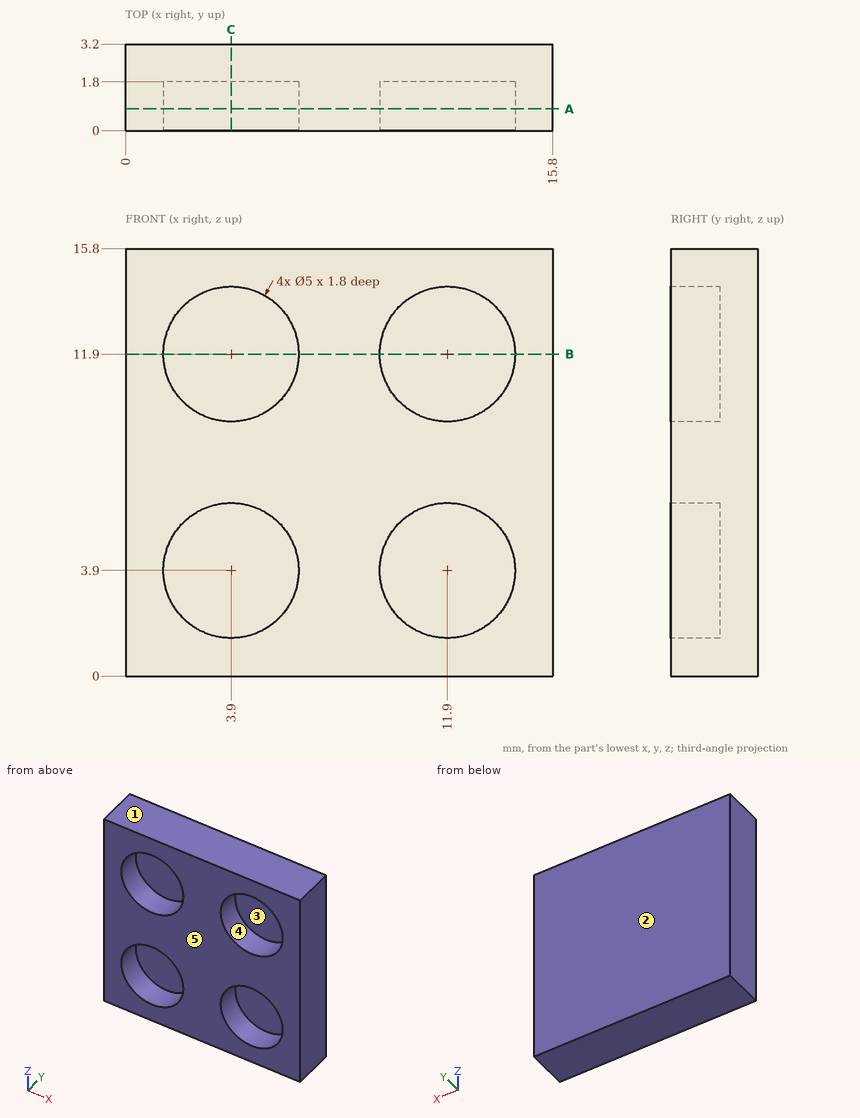
Study the drawing (mm; zero at the part's minimum x, y, z) and answer. A direction names the side the tool comes from. Round coordinates to 2 decimals unless told otherwise and drop trailing zeros. Loops run counter-clockwise (first coordinate to the right, second up) from the corner with the lowest first, then second, coordinate; pieces in that order, holes last.
Q1. Which of the six approach directions +Z, -Z, +X, -X, +Y, -Y give full straight-line access (tool end or side, diameter ignored) to the marked faces 4 and 5?
Q2. Given pin 1 Ø1.5 at (x, z) = (12, 13) entering from -Y, flat-ended and moving along its own axis, determine where the tip first touches the part or whether it passes through.
Q3. Find the intervals of material crossed by line 1 (X direction, y = 1, z = 11.9); line 2 (X direction, y = 1.4, z = 13) (3 decimals), in increasing order.
Q4. Section C-C, the plane x = 3.9 is taken. Determine the outline of the cut face in (y, z).
Q5. For a pull along Z with two mould halves and no side action, classify the marked faces 1, 2 and 3 as released by +Z, released by -Z, zero draft, split by the parting line, or undercut.
Q6. Section B-B, the plane z = 11.9 is taken. Determine the outline of the cut face in (x, y).
Q7. Section A-A, the plane y = 0.8 is taken. Determine the outline of the cut face in (x, z), then the cut area to 3 significant figures.
Completed:
1. face 4: -Y
1. face 5: +Z, -Z, +X, -X, -Y
2. pin 1: stops at y = 1.8
3. line 1: x = 0 to 1.4, 6.4 to 9.4, 14.4 to 15.8
3. line 2: x = 0 to 1.655, 6.145 to 9.655, 14.145 to 15.8
4. outline: (0, 0) - (3.2, 0) - (3.2, 15.8) - (0, 15.8) - (0, 14.4) - (1.8, 14.4) - (1.8, 9.4) - (0, 9.4) - (0, 6.4) - (1.8, 6.4) - (1.8, 1.4) - (0, 1.4) - close
5. face 1: released by +Z
5. face 2: zero draft
5. face 3: undercut
6. outline: (0, 0) - (1.4, 0) - (1.4, 1.8) - (6.4, 1.8) - (6.4, 0) - (9.4, 0) - (9.4, 1.8) - (14.4, 1.8) - (14.4, 0) - (15.8, 0) - (15.8, 3.2) - (0, 3.2) - close
7. outline: (0, 0) - (15.8, 0) - (15.8, 15.8) - (0, 15.8) - close; hole circle Ø5 at (3.9, 3.9); hole circle Ø5 at (3.9, 11.9); hole circle Ø5 at (11.9, 3.9); hole circle Ø5 at (11.9, 11.9)
7. area: 171 mm2
